from build123d import *

# Parameters (mm, degrees)
ESBO_O1_W                = 15.8
ESBO_O1_H                = 100
RESSALTO_EXTRUS_O1_DEPTH = 1.68
ESBO_O3_W                = 1.68
ESBO_O3_H                = 100
RESSALTO_EXTRUS_O2_DEPTH = 15.8
ESBO_O4_R                = 1.5
CORTE_EXTRUS_O1_DEPTH    = 103.493535406
ESBO_O5_R                = 1.5
CORTE_EXTRUS_O2_DEPTH    = 103.465994359


with BuildPart() as part:
    # Esboço1 → Ressalto-extrusão1 (new body)
    with BuildSketch(Plane.XY):
        with Locations((-7.9, 50)):
            Rectangle(ESBO_O1_W, ESBO_O1_H)
    extrude(amount=RESSALTO_EXTRUS_O1_DEPTH)

    # Esboço3 → Ressalto-extrusão2 (add)
    with BuildSketch(Plane.XY.offset(1.68)):
        with Locations((-0.84, 50)):
            Rectangle(ESBO_O3_W, ESBO_O3_H)
    extrude(amount=RESSALTO_EXTRUS_O2_DEPTH)

    # Esboço4 → Corte-extrusão1 (cut, through all)
    with BuildSketch(Plane.ZY.offset(1.68)):
        with Locations((11, 94)):
            Circle(ESBO_O4_R)
        with Locations((11, 6)):
            Circle(ESBO_O4_R)
    extrude(amount=-CORTE_EXTRUS_O1_DEPTH, mode=Mode.SUBTRACT)

    # Esboço5 → Corte-extrusão2 (cut, through all)
    with BuildSketch(Plane.XY.offset(1.68)):
        with Locations((-11, 94)):
            Circle(ESBO_O5_R)
        with Locations((-11, 6)):
            Circle(ESBO_O5_R)
    extrude(amount=-CORTE_EXTRUS_O2_DEPTH, mode=Mode.SUBTRACT)


solid = part.part
Could you check a few things on this model? Use its own coordinates, in mm. A direction names the side the tool comes from. Coordinates: 2 decimals unless noted, no trailing zeros. Loops run counter-clockwise (first coordinate to the right, second up) from the corner with the lowest first, then second, coordinate; pieces in that order, holes last. Notation, with made-up numbers: (65.5, 42.25) -> (114.5, 42.25) arc R6 ccw to (114.5, 53.25) -> close; hole circle Ø9 at (-25, -8.5). An arc over 180 degrees is marked (long way). Answer in a Markdown table with one row per item.
(1) Imagine slicing it at C-C (x = -11). List the corners of the cut face in (y, z) for me.
Results found:
| item | result |
|---|---|
| outline | (0, 0) -> (4.5, 0) -> (4.5, 1.68) -> (0, 1.68) -> close; (7.5, 0) -> (92.5, 0) -> (92.5, 1.68) -> (7.5, 1.68) -> close; (95.5, 0) -> (100, 0) -> (100, 1.68) -> (95.5, 1.68) -> close |
(2) Will these pins go through, and if not, where does the flat tip stop? pin 1 Ø4.5 at (y, z) = (37.5, 13) entering from -X; pin 2 Ø3.5 at (x, y) = (-11, 94) entering from +Z.
Results found:
| item | result |
|---|---|
| pin 1 | stops at x = -1.68 |
| pin 2 | stops at z = 1.68 |
(3) Thinking about a two-plate mould opening in Z: for faces 3 (the face through (-15.8, 49, 1)), 4 (the face through (-0.852, 95.487, 10.805)), 5 (the face through (-8, 51, 0)), which applies, released by +Z, released by -Z, zero draft, split by the parting line, or undercut?
Results found:
| item | result |
|---|---|
| face 3 | zero draft |
| face 4 | undercut |
| face 5 | released by -Z |
(4) For faces 1 (the face through (-1.68, 49, 9)), 2 (the face through (-1, 100, 5)), which set-ups out of +Z, -Z, +X, -X, +Y, -Y let a thin tool reach every point of the face, with its end or its side?
Results found:
| item | result |
|---|---|
| face 1 | +Z, -X, +Y, -Y |
| face 2 | +Z, -Z, +X, -X, +Y |
(5) Imagine slicing it at A-A (y = 6). List the corners of the cut face in (x, z) for me.
Results found:
| item | result |
|---|---|
| outline | (-15.8, 0) -> (-12.5, 0) -> (-12.5, 1.68) -> (-15.8, 1.68) -> close; (-9.5, 0) -> (0, 0) -> (0, 9.5) -> (-1.68, 9.5) -> (-1.68, 1.68) -> (-9.5, 1.68) -> close; (-1.68, 12.5) -> (0, 12.5) -> (0, 17.48) -> (-1.68, 17.48) -> close |
(6) Imagine slicing it at B-B (z = 11). List the corners of the cut face in (x, y) for me, plus the area to 3 significant figures.
Results found:
| item | result |
|---|---|
| outline | (-1.68, 0) -> (0, 0) -> (0, 4.5) -> (-1.68, 4.5) -> close; (-1.68, 7.5) -> (0, 7.5) -> (0, 92.5) -> (-1.68, 92.5) -> close; (-1.68, 95.5) -> (0, 95.5) -> (0, 100) -> (-1.68, 100) -> close |
| area | 158 mm^2 |
(7) Imagine slicing it at D-D (y = 37). List the corners of the cut face in (x, z) for me.
Results found:
| item | result |
|---|---|
| outline | (-15.8, 0) -> (0, 0) -> (0, 17.48) -> (-1.68, 17.48) -> (-1.68, 1.68) -> (-15.8, 1.68) -> close |
(8) If I drill on probe 1 along Y at (x, z) = (-0.4, 11); probe 2 along Z at (x, y) = (-0.75, 94); probe 3 along X at (y, z) = (94, 0.8), over which ranges is the centre line in solid material (lowest first)?
Results found:
| item | result |
|---|---|
| probe 1 | y = 0 to 4.5, 7.5 to 92.5, 95.5 to 100 |
| probe 2 | z = 0 to 9.5, 12.5 to 17.48 |
| probe 3 | x = -15.8 to -12.5, -9.5 to 0 |
